CAD build for the part. Positions are in the model's coordinates, mm. Face numbers are marked on the shaded views. Coordinates: 2 decimals unless noted, no trailing zeros. Loops run counter-clockwise (first coordinate to the right, second up) from the corner with the lowest first, then second, coordinate; pieces in that order, holes last. Notation, with made-up numbers: (-11, 6.5) -> (0, 6.5) arc R29 cw to (0, 38.5) -> close; hole circle Ø5 at (33.25, 9.5). An arc over 180 degrees is marked (long way). Return JSON: item names as keys, results as strings. Group by question number.
(1) Saw through at B-B on z = 17.75. Write the cut outline in (x, y).
(2) Probe L1, parallel to Y at x = 0, z = 5.75; L2, parallel to Y at x = 6.5, z = 8.5; L3, parallel to X at y = 4, z = 7.5. List the from-to ranges inside material, lowest first.
(3) Mould opens along Y. For the marked faces 1, 2 and 3 say: pulls with the +Y half, pulls with the -Y half, needs draft (parallel to the pull), parting line crosses it, or undercut.
(4) Saw through at A-A on z = 6.5. Write the cut outline in (x, y).
(5) Flat gauge pins, fed straight in: pin 1 Ø3 at (x, y) = (1.5, -6.5) entering from -Z; pin 2 Ø5 at (x, y) = (-3, 4) entering from -Z; pin 3 Ø5 at (y, z) = (-10, 8.5) entering from +X; pin 4 Ø6 at (x, y) = (0, 14) entering from +Z. Where does each tip first touch, or does it go through?
```python
from build123d import *


with BuildPart() as f1:
    # F0 (on Front) → F1 (revolve)
    with BuildSketch(Plane.XZ):
        with BuildLine():
            Line((-8.1026, 9.672707), (0, 9.672707))
            Line((0, 9.672707), (0, 27.15264))
            ThreePointArc((0, 27.15264), (-10.249929, 26.01392), (-20, 22.65329))
            Line((-20, 22.65329), (-20, 20.65329))
            Line((-20, 20.65329), (-16.129, 16.78229))
            ThreePointArc((-16.129, 16.78229), (-15.25032, 14.66097), (-16.129, 12.539649))
            Line((-16.129, 12.539649), (-16.129, 0))
            Line((-16.129, 0), (-8.1026, 0))
            Line((-8.1026, 0), (-8.1026, 9.672707))
        make_face()
    revolve(axis=Axis((0, 0, 16.521212), (0, 0, 1)))


solid = f1.part
```
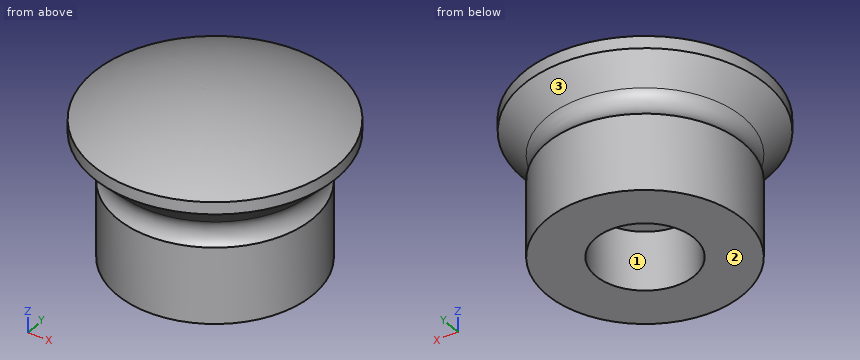
Geometry results:
{
 "1": {"outline": "circle Ø34.19 at (0, 0)"},
 "2": {"L1": "-16.13 to -8.1, 8.1 to 16.13", "L2": "-14.76 to -4.84, 4.84 to 14.76", "L3": "-15.63 to -7.05, 7.05 to 15.63"},
 "3": {"face 1": "undercut", "face 2": "needs draft", "face 3": "parting line crosses it"},
 "4": {"outline": "circle Ø32.26 at (0, 0); hole circle Ø16.21 at (0, 0)"},
 "5": {"pin 1": "z = 0", "pin 2": "z = 9.67", "pin 3": "x = 14.28", "pin 4": "z = 25.84"}
}
